For this review, take the finished solid that the model builds, in its own axes (mm). Coordinates: 2 decimals unless noted, no trailing zeros. One line per question, with ' | ' between items.
from build123d import *

# Parameters (mm, degrees)
SKETCH_1_W          = 330
SKETCH_1_H          = 178
EXTRUDE_1_DEPTH     = 2
CUT_EXTRUDE_1_REACH = 189.483
CUT_EXTRUDE_2_REACH = 189.483
SKETCH_3_R          = 1.6
CUT_EXTRUDE_4_DEPTH = 188.483332593
FILLET_1_R          = 1


with BuildPart() as part:
    # 草图1 → 凸台-拉伸1 (new body)
    with BuildSketch(Plane.XY):
        Rectangle(SKETCH_1_W, SKETCH_1_H)
    extrude(amount=EXTRUDE_1_DEPTH)

    # 草图2 → 切除-拉伸1 (cut, up to next)
    with BuildSketch(Plane.XY.offset(2), mode=Mode.PRIVATE) as cut_extrude_1_sk1:
        with BuildLine():
            Line((65, 15), (145, 15))
            ThreePointArc((145, 15), (149, 11), (145, 7))
            Line((145, 7), (65, 7))
            ThreePointArc((65, 7), (61, 11), (65, 15))
        make_face()
    cut_extrude_1_tool1 = extrude(cut_extrude_1_sk1.sketch, amount=-CUT_EXTRUDE_1_REACH, mode=Mode.PRIVATE) & part.part
    # 草图2 → 切除-拉伸1 (cut, up to next)
    with BuildSketch(Plane.XY.offset(2), mode=Mode.PRIVATE) as cut_extrude_1_sk2:
        with BuildLine():
            Line((65, -4.428571429), (145, -4.428571429))
            ThreePointArc((145, -4.428571429), (149, -0.428571429), (145, 3.571428571))
            Line((145, 3.571428571), (65, 3.571428571))
            ThreePointArc((65, 3.571428571), (61, -0.428571429), (65, -4.428571429))
        make_face()
    cut_extrude_1_tool2 = extrude(cut_extrude_1_sk2.sketch, amount=-CUT_EXTRUDE_1_REACH, mode=Mode.PRIVATE) & part.part
    # 草图2 → 切除-拉伸1 (cut, up to next)
    with BuildSketch(Plane.XY.offset(2), mode=Mode.PRIVATE) as cut_extrude_1_sk3:
        with BuildLine():
            Line((65, -15.857142857), (145, -15.857142857))
            ThreePointArc((145, -15.857142857), (149, -11.857142857), (145, -7.857142857))
            Line((145, -7.857142857), (65, -7.857142857))
            ThreePointArc((65, -7.857142857), (61, -11.857142857), (65, -15.857142857))
        make_face()
    cut_extrude_1_tool3 = extrude(cut_extrude_1_sk3.sketch, amount=-CUT_EXTRUDE_1_REACH, mode=Mode.PRIVATE) & part.part
    # 草图2 → 切除-拉伸1 (cut, up to next)
    with BuildSketch(Plane.XY.offset(2), mode=Mode.PRIVATE) as cut_extrude_1_sk4:
        with BuildLine():
            Line((65, -27.285714286), (145, -27.285714286))
            ThreePointArc((145, -27.285714286), (149, -23.285714286), (145, -19.285714286))
            Line((145, -19.285714286), (65, -19.285714286))
            ThreePointArc((65, -19.285714286), (61, -23.285714286), (65, -27.285714286))
        make_face()
    cut_extrude_1_tool4 = extrude(cut_extrude_1_sk4.sketch, amount=-CUT_EXTRUDE_1_REACH, mode=Mode.PRIVATE) & part.part
    # 草图2 → 切除-拉伸1 (cut, up to next)
    with BuildSketch(Plane.XY.offset(2), mode=Mode.PRIVATE) as cut_extrude_1_sk5:
        with BuildLine():
            Line((65, -38.714285714), (145, -38.714285714))
            ThreePointArc((145, -38.714285714), (149, -34.714285714), (145, -30.714285714))
            Line((145, -30.714285714), (65, -30.714285714))
            ThreePointArc((65, -30.714285714), (61, -34.714285714), (65, -38.714285714))
        make_face()
    cut_extrude_1_tool5 = extrude(cut_extrude_1_sk5.sketch, amount=-CUT_EXTRUDE_1_REACH, mode=Mode.PRIVATE) & part.part
    # 草图2 → 切除-拉伸1 (cut, up to next)
    with BuildSketch(Plane.XY.offset(2), mode=Mode.PRIVATE) as cut_extrude_1_sk6:
        with BuildLine():
            Line((65, -50.142857143), (145, -50.142857143))
            ThreePointArc((145, -50.142857143), (149, -46.142857143), (145, -42.142857143))
            Line((145, -42.142857143), (65, -42.142857143))
            ThreePointArc((65, -42.142857143), (61, -46.142857143), (65, -50.142857143))
        make_face()
    cut_extrude_1_tool6 = extrude(cut_extrude_1_sk6.sketch, amount=-CUT_EXTRUDE_1_REACH, mode=Mode.PRIVATE) & part.part
    # 草图2 → 切除-拉伸1 (cut, up to next)
    with BuildSketch(Plane.XY.offset(2), mode=Mode.PRIVATE) as cut_extrude_1_sk7:
        with BuildLine():
            Line((65, -61.571428571), (145, -61.571428571))
            ThreePointArc((145, -61.571428571), (149, -57.571428571), (145, -53.571428571))
            Line((145, -53.571428571), (65, -53.571428571))
            ThreePointArc((65, -53.571428571), (61, -57.571428571), (65, -61.571428571))
        make_face()
    cut_extrude_1_tool7 = extrude(cut_extrude_1_sk7.sketch, amount=-CUT_EXTRUDE_1_REACH, mode=Mode.PRIVATE) & part.part
    # 草图2 → 切除-拉伸1 (cut, up to next)
    with BuildSketch(Plane.XY.offset(2), mode=Mode.PRIVATE) as cut_extrude_1_sk8:
        with BuildLine():
            Line((65, -73), (145, -73))
            ThreePointArc((145, -73), (149, -69), (145, -65))
            Line((145, -65), (65, -65))
            ThreePointArc((65, -65), (61, -69), (65, -73))
        make_face()
    cut_extrude_1_tool8 = extrude(cut_extrude_1_sk8.sketch, amount=-CUT_EXTRUDE_1_REACH, mode=Mode.PRIVATE) & part.part
    add(cut_extrude_1_tool1.solids().sort_by_distance((105, 11, 2))[0], mode=Mode.SUBTRACT)
    add(cut_extrude_1_tool2.solids().sort_by_distance((105, -0.428571, 2))[0], mode=Mode.SUBTRACT)
    add(cut_extrude_1_tool3.solids().sort_by_distance((105, -11.857143, 2))[0], mode=Mode.SUBTRACT)
    add(cut_extrude_1_tool4.solids().sort_by_distance((105, -23.285714, 2))[0], mode=Mode.SUBTRACT)
    add(cut_extrude_1_tool5.solids().sort_by_distance((105, -34.714286, 2))[0], mode=Mode.SUBTRACT)
    add(cut_extrude_1_tool6.solids().sort_by_distance((105, -46.142857, 2))[0], mode=Mode.SUBTRACT)
    add(cut_extrude_1_tool7.solids().sort_by_distance((105, -57.571429, 2))[0], mode=Mode.SUBTRACT)
    add(cut_extrude_1_tool8.solids().sort_by_distance((105, -69, 2))[0], mode=Mode.SUBTRACT)

    # 草图3 → 切除-拉伸2 (cut, up to next)
    with BuildSketch(Plane.XY.offset(2), mode=Mode.PRIVATE) as cut_extrude_2_sk1:
        with Locations((-162, 51)):
            Circle(SKETCH_3_R)
    cut_extrude_2_tool1 = extrude(cut_extrude_2_sk1.sketch, amount=-CUT_EXTRUDE_2_REACH, mode=Mode.PRIVATE) & part.part
    # 草图3 → 切除-拉伸2 (cut, up to next)
    with BuildSketch(Plane.XY.offset(2), mode=Mode.PRIVATE) as cut_extrude_2_sk2:
        with Locations((-162, 31)):
            Circle(SKETCH_3_R)
    cut_extrude_2_tool2 = extrude(cut_extrude_2_sk2.sketch, amount=-CUT_EXTRUDE_2_REACH, mode=Mode.PRIVATE) & part.part
    # 草图3 → 切除-拉伸2 (cut, up to next)
    with BuildSketch(Plane.XY.offset(2), mode=Mode.PRIVATE) as cut_extrude_2_sk3:
        with Locations((-160, -81)):
            Circle(SKETCH_3_R)
    cut_extrude_2_tool3 = extrude(cut_extrude_2_sk3.sketch, amount=-CUT_EXTRUDE_2_REACH, mode=Mode.PRIVATE) & part.part
    # 草图3 → 切除-拉伸2 (cut, up to next)
    with BuildSketch(Plane.XY.offset(2), mode=Mode.PRIVATE) as cut_extrude_2_sk4:
        with Locations((145, -81)):
            Circle(SKETCH_3_R)
    cut_extrude_2_tool4 = extrude(cut_extrude_2_sk4.sketch, amount=-CUT_EXTRUDE_2_REACH, mode=Mode.PRIVATE) & part.part
    # 草图3 → 切除-拉伸2 (cut, up to next)
    with BuildSketch(Plane.XY.offset(2), mode=Mode.PRIVATE) as cut_extrude_2_sk5:
        with Locations((125, -81)):
            Circle(SKETCH_3_R)
    cut_extrude_2_tool5 = extrude(cut_extrude_2_sk5.sketch, amount=-CUT_EXTRUDE_2_REACH, mode=Mode.PRIVATE) & part.part
    # 草图3 → 切除-拉伸2 (cut, up to next)
    with BuildSketch(Plane.XY.offset(2), mode=Mode.PRIVATE) as cut_extrude_2_sk6:
        with Locations((160, 86)):
            Circle(SKETCH_3_R)
    cut_extrude_2_tool6 = extrude(cut_extrude_2_sk6.sketch, amount=-CUT_EXTRUDE_2_REACH, mode=Mode.PRIVATE) & part.part
    add(cut_extrude_2_tool1.solids().sort_by_distance((-162, 51, 2))[0], mode=Mode.SUBTRACT)
    add(cut_extrude_2_tool2.solids().sort_by_distance((-162, 31, 2))[0], mode=Mode.SUBTRACT)
    add(cut_extrude_2_tool3.solids().sort_by_distance((-160, -81, 2))[0], mode=Mode.SUBTRACT)
    add(cut_extrude_2_tool4.solids().sort_by_distance((145, -81, 2))[0], mode=Mode.SUBTRACT)
    add(cut_extrude_2_tool5.solids().sort_by_distance((125, -81, 2))[0], mode=Mode.SUBTRACT)
    add(cut_extrude_2_tool6.solids().sort_by_distance((160, 86, 2))[0], mode=Mode.SUBTRACT)

    # 草图5 → 切除-拉伸4 (cut, through all)
    with BuildSketch(Plane.XY.offset(2)):
        with BuildLine():
            Line((167, 52), (167, 24))
            ThreePointArc((167, 24), (165, 22), (163, 24))
            Line((163, 24), (163, 52))
            ThreePointArc((163, 52), (165, 54), (167, 52))
        make_face()
    extrude(amount=-CUT_EXTRUDE_4_DEPTH, mode=Mode.SUBTRACT)

    # 圆角1
    fillet_1_edges = [part.edges().sort_by_distance(p)[0] for p in [
        (165, 54, 1),
        (165, 22, 1),
    ]]
    fillet(fillet_1_edges, radius=FILLET_1_R)


solid = part.part
1) To check wall thickness, follow line 1 along X through (y, z) = (-81, 0.8); line 2 along X through (y, z) = (86, 0.85); line 3 along X through (y, z) = (-23.5, 1.1). State the ranges of each line that lie inside material, in increasing order. Write a range as [from, to].
Responses:
line 1: [-165, -161.6], [-158.4, 123.4], [126.6, 143.4], [146.6, 165] | line 2: [-165, 158.4], [161.6, 165] | line 3: [-165, 61.01], [148.99, 165]
2) We need section A-A on z = 0.8. State how many separate pieces and enclosed holes the cut face has, then the cut area to 3 significant figures.
Responses:
separate pieces: 1 | enclosed holes: 14 | area: 53,100 mm^2
3) Insertion check: pin 1 Ø10 at (x, y) = (-84.5, 34) entering from -Z. The pin has a flat end and moves straight along its axis. Give the tip position at first contact, or say it passes through.
Responses:
pin 1: z = 0
